Here's how the part is built. I have some questions about the finished solid (model axes, mm). Give positions to 0.01 mm unless a question says otherwise; leave off trailing zeros. Loops run counter-clockwise (first coordinate to the right, second up) from the corner with the lowest first, then second, coordinate; pieces in that order, holes last.
Q1. If we section it at B-B (y = 10): Please give me the cut outline in (x, z), plus the area to 3 significant figures.
Q2. I need wall thicknesses on line 1 (Y direction, x = 35, z = 25.9); line 2 (Y direction, x = 36.5, z = 26.8); line 3 (X direction, y = 12, z = 26.85). Which ranges of each line are inside material? Lowest first, please.
Q3. If we section it at C-C (z = 25.5): Please give me the cut outline in (x, y), plus the area to 3 significant figures.
Q4. Will this pin go through, and if not, where does the flat tip stop? P1, Ø3, axis at x = 35, y = 90, coming from the +Z side.
Q5. If we section it at A-A (x = 35): Please give me the cut outline in (y, z).
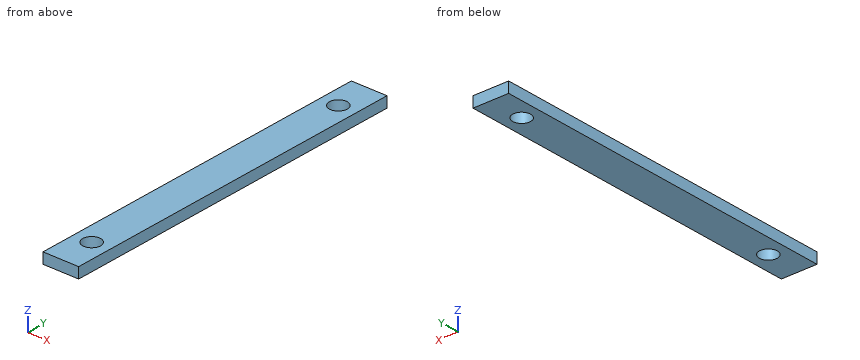
from build123d import *

# Parameters (mm, degrees)
CYLINDER010_R     = 2.5
CYLINDER010_DEPTH = 3
CYLINDER009_R     = 2.5
CYLINDER009_DEPTH = 3
BOX002_W          = 10
BOX002_H          = 100
BOX002_DEPTH      = 3


with BuildPart() as cylinder010:
    # Cylinder010 → Cylinder010 (new body)
    with BuildSketch(Plane(origin=(35, 90, 24.5), x_dir=(1, 0, 0), z_dir=(0, 0, 1))):
        Circle(CYLINDER010_R)
    extrude(amount=CYLINDER010_DEPTH)


with BuildPart() as cylinder009:
    # Cylinder009 → Cylinder009 (new body)
    with BuildSketch(Plane(origin=(35, 10, 24.5), x_dir=(1, 0, 0), z_dir=(0, 0, 1))):
        Circle(CYLINDER009_R)
    extrude(amount=CYLINDER009_DEPTH)


with BuildPart() as cut_1st_support_bar:
    # Box002 → Box002 (new body)
    with BuildSketch(Plane(origin=(30, 0, 24.5), x_dir=(1, 0, 0), z_dir=(0, 0, 1))):
        with Locations((5, 50)):
            Rectangle(BOX002_W, BOX002_H)
    extrude(amount=BOX002_DEPTH)

    # Cut003: cut Cylinder009
    add(cylinder009.part, mode=Mode.SUBTRACT)

    # Cut004: cut Cylinder010
    add(cylinder010.part, mode=Mode.SUBTRACT)


solid = cut_1st_support_bar.part
Check sheet entries:
1. outline: (30, 24.5) - (32.5, 24.5) - (32.5, 27.5) - (30, 27.5) - close; (37.5, 24.5) - (40, 24.5) - (40, 27.5) - (37.5, 27.5) - close
1. area: 15.0 mm2
2. line 1: y = 0 to 7.5, 12.5 to 87.5, 92.5 to 100
2. line 2: y = 0 to 8, 12 to 88, 92 to 100
2. line 3: x = 30 to 33.5, 36.5 to 40
3. outline: (30, 0) - (40, 0) - (40, 100) - (30, 100) - close; hole circle Ø5 at (35, 10); hole circle Ø5 at (35, 90)
3. area: 961 mm2
4. P1: passes through
5. outline: (0, 24.5) - (7.5, 24.5) - (7.5, 27.5) - (0, 27.5) - close; (12.5, 24.5) - (87.5, 24.5) - (87.5, 27.5) - (12.5, 27.5) - close; (92.5, 24.5) - (100, 24.5) - (100, 27.5) - (92.5, 27.5) - close
